Design review of the part built by this model. Coordinates are the model's own, in mm. Face numbers are marked on the shaded views. A direction names the side the tool comes from. Round coordinates to 2 decimals unless told otherwise and drop trailing zeros. Order: outer loops, then holes, each group sorted by start corner. A loop starts at its lowest first (then second) coordinate and runs counter-clockwise, first axis right, second up. Notation, with made-up numbers: M 31.25,61 L 67.25,61 A25 cw 67.25,90 Z; hole C -22,0 d7. An arc over 180 degrees is marked long. Use a Markdown table: item, result. Add a question column.
(1) Take a section at D-D (z = -10). Write out the cut boundary in (x, y) (1 decimal).
(2) To check wall thickness, follow probe 1 along Z at (x, y) = (1.25, 4); probe 2 along X at (y, z) = (-5.5, -14); probe 3 along Y at (x, z) = (-6, 2). State the ranges of each line that lie inside material, in increasing order. Write a range as from..to.
(3) For pin 1 (4 mm diameter, centred on x = -6.5, z = -4.5, fed in from -Y); pin 2 (1 mm diameter, centred on y = -6, z = -17.5, fed in from -X); pin 3 (2 mm diameter, centred on y = -4.5, z = -16, fed in from +X), all flat-tipped, find the tip position at first contact; note any pin that passes through.
(4) Take a section at A-A (y = 0). Write out the cut boundary in (x, z).
(5) Take a section at C-C (z = 0.5). Write out the cut boundary in (x, y).
(6) Machinability: for the marked faces 1 and 2, which of the approach directions +Z, -Z, +X, -X, +Y, -Y give a long, thin tool a straight path to every point of the face, cutting with its end or side? Answer none if there is none.
(7) Take a section at B-B (x = -3). Write out the cut boundary in (y, z), then the cut area to 3 significant figures.
Autodesk Inventor part; units mm, degrees
ref_plane "YZ Plane" through (0, 0, 0) normal (1, 0, 0) x (0, 1, 0)
ref_plane "XZ Plane" through (0, 0, 0) normal (0, 1, 0) x (-1, 0, 0)
ref_plane "XY Plane" through (0, 0, 0) normal (0, 0, 1) x (1, 0, 0)
sketch "Sketch1" plane through (0, 0, 0) normal (0, 0, 1) x (1, 0, 0)
  circle A0 centre (-0.6115, -1.5992) radius 4.7625
  line L0 (-7.9438, -1.5992) -> (-4.2777, 4.7508)
  line L1 (-4.2777, 4.7508) -> (3.0547, 4.7508)
  line L2 (3.0547, 4.7508) -> (6.7209, -1.5992)
  line L3 (6.7209, -1.5992) -> (3.0547, -7.9492)
  line L4 (3.0547, -7.9492) -> (-4.2777, -7.9492)
  line L5 (-4.2777, -7.9492) -> (-7.9438, -1.5992)
  dimension "d10" = 12.7
  dimension "d20" = 9.525
extrude "Extrusion1" add sketch "Sketch1" against normal blind 25.4 contours A0
extrude "Extrusion2" add sketch "Sketch1" along normal blind 5.08 contours A0 | L0 L1 L2 L3 L4 L5
thread "Thread2"
properties part number "HW-00043"
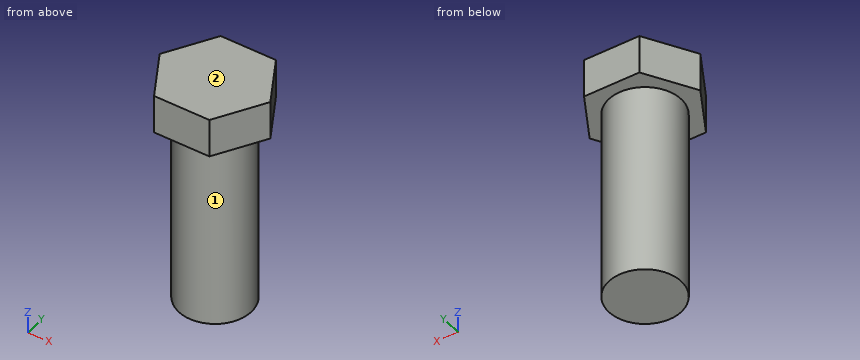
Verdict:
| question | item | result |
|---|---|---|
| 1 | outline | C -0.6,-1.6 d9.5 |
| 2 | probe 1 | z = 0..5.08 |
| 2 | probe 2 | x = -3.34..2.12 |
| 2 | probe 3 | y = -4.97..1.77 |
| 3 | pin 1 | stops at y = -4.35 |
| 3 | pin 2 | stops at x = -3.34 |
| 3 | pin 3 | stops at x = 3.76 |
| 4 | outline | M -7.02,0 L -5.1,0 L -5.1,-25.4 L 3.87,-25.4 L 3.87,0 L 5.8,0 L 5.8,5.08 L -7.02,5.08 Z |
| 5 | outline | M -7.94,-1.6 L -4.28,-7.95 L 3.05,-7.95 L 6.72,-1.6 L 3.05,4.75 L -4.28,4.75 Z |
| 6 | face 1 | -Z |
| 6 | face 2 | +Z, +X, -X, +Y, -Y |
| 7 | outline | M -7.95,0 L -5.72,0 L -5.72,-25.4 L 2.52,-25.4 L 2.52,0 L 4.75,0 L 4.75,5.08 L -7.95,5.08 Z |
| 7 | area | 274 mm^2 |
